```python
from build123d import *

# Parameters (mm, degrees)
SKETCH069_W                  = 20.5
SKETCH069_H                  = 15
PAD036_DEPTH                 = 1.5
SKETCH071_W                  = 0.6
SKETCH071_H                  = 0.6
PAD037_DEPTH                 = 8
SKETCH071_LINEARPATTERN_2_W  = 0.6
SKETCH071_LINEARPATTERN_2_H  = 0.6
PAD037_LINEARPATTERN_2_DEPTH = 8
SKETCH071_LINEARPATTERN_3_W  = 0.6
SKETCH071_LINEARPATTERN_3_H  = 0.6
PAD037_LINEARPATTERN_3_DEPTH = 8
SKETCH071_LINEARPATTERN_4_W  = 0.6
SKETCH071_LINEARPATTERN_4_H  = 0.6
PAD037_LINEARPATTERN_4_DEPTH = 8
SKETCH071_LINEARPATTERN_5_W  = 0.6
SKETCH071_LINEARPATTERN_5_H  = 0.6
PAD037_LINEARPATTERN_5_DEPTH = 8
SKETCH071_LINEARPATTERN_6_W  = 0.6
SKETCH071_LINEARPATTERN_6_H  = 0.6
PAD037_LINEARPATTERN_6_DEPTH = 8
SKETCH071_LINEARPATTERN_7_W  = 0.6
SKETCH071_LINEARPATTERN_7_H  = 0.6
PAD037_LINEARPATTERN_7_DEPTH = 8
SKETCH071_LINEARPATTERN_8_W  = 0.6
SKETCH071_LINEARPATTERN_8_H  = 0.6
PAD037_LINEARPATTERN_8_DEPTH = 8
SKETCH070_W                  = 20.5
SKETCH070_H                  = 2.5
PAD038_DEPTH                 = 2
SKETCH074_W                  = 1.239915
SKETCH074_H                  = 2.350915
SKETCH074_W_2                = 6.389756
SKETCH074_H_2                = 4.341472
PAD040_DEPTH                 = 0.5


with BuildPart() as part:
    # Sketch069 → Pad036 (new body)
    with BuildSketch(Plane.XY.offset(2)):
        Rectangle(SKETCH069_W, SKETCH069_H)
    extrude(amount=PAD036_DEPTH)

    # Sketch071 → Pad037 (join)
    with BuildSketch(Plane(origin=(-9.5, -6.2, 2), x_dir=(1, 0, 0), z_dir=(0, 0, 1))):
        Rectangle(SKETCH071_W, SKETCH071_H)
    pad037 = extrude(amount=-PAD037_DEPTH)

    # Sketch071 LinearPattern 2 → Pad037 LinearPattern 2 (add)
    with BuildSketch(Plane(origin=(-6.871429, -6.2, 2), x_dir=(1, 0, 0), z_dir=(0, 0, 1))):
        Rectangle(SKETCH071_LINEARPATTERN_2_W, SKETCH071_LINEARPATTERN_2_H)
    pad037_linearpattern_2 = extrude(amount=-PAD037_LINEARPATTERN_2_DEPTH)

    # Sketch071 LinearPattern 3 → Pad037 LinearPattern 3 (add)
    with BuildSketch(Plane(origin=(-4.242857, -6.2, 2), x_dir=(1, 0, 0), z_dir=(0, 0, 1))):
        Rectangle(SKETCH071_LINEARPATTERN_3_W, SKETCH071_LINEARPATTERN_3_H)
    pad037_linearpattern_3 = extrude(amount=-PAD037_LINEARPATTERN_3_DEPTH)

    # Sketch071 LinearPattern 4 → Pad037 LinearPattern 4 (add)
    with BuildSketch(Plane(origin=(-1.614286, -6.2, 2), x_dir=(1, 0, 0), z_dir=(0, 0, 1))):
        Rectangle(SKETCH071_LINEARPATTERN_4_W, SKETCH071_LINEARPATTERN_4_H)
    pad037_linearpattern_4 = extrude(amount=-PAD037_LINEARPATTERN_4_DEPTH)

    # Sketch071 LinearPattern 5 → Pad037 LinearPattern 5 (add)
    with BuildSketch(Plane(origin=(1.014286, -6.2, 2), x_dir=(1, 0, 0), z_dir=(0, 0, 1))):
        Rectangle(SKETCH071_LINEARPATTERN_5_W, SKETCH071_LINEARPATTERN_5_H)
    pad037_linearpattern_5 = extrude(amount=-PAD037_LINEARPATTERN_5_DEPTH)

    # Sketch071 LinearPattern 6 → Pad037 LinearPattern 6 (add)
    with BuildSketch(Plane(origin=(3.642857, -6.2, 2), x_dir=(1, 0, 0), z_dir=(0, 0, 1))):
        Rectangle(SKETCH071_LINEARPATTERN_6_W, SKETCH071_LINEARPATTERN_6_H)
    pad037_linearpattern_6 = extrude(amount=-PAD037_LINEARPATTERN_6_DEPTH)

    # Sketch071 LinearPattern 7 → Pad037 LinearPattern 7 (add)
    with BuildSketch(Plane(origin=(6.271429, -6.2, 2), x_dir=(1, 0, 0), z_dir=(0, 0, 1))):
        Rectangle(SKETCH071_LINEARPATTERN_7_W, SKETCH071_LINEARPATTERN_7_H)
    pad037_linearpattern_7 = extrude(amount=-PAD037_LINEARPATTERN_7_DEPTH)

    # Sketch071 LinearPattern 8 → Pad037 LinearPattern 8 (add)
    with BuildSketch(Plane(origin=(8.9, -6.2, 2), x_dir=(1, 0, 0), z_dir=(0, 0, 1))):
        Rectangle(SKETCH071_LINEARPATTERN_8_W, SKETCH071_LINEARPATTERN_8_H)
    pad037_linearpattern_8 = extrude(amount=-PAD037_LINEARPATTERN_8_DEPTH)

    # Mirrored: Pad037, Pad037 LinearPattern 2, Pad037 LinearPattern 3, Pad037 LinearPattern 4, Pad037 LinearPattern 5, Pad037 LinearPattern 6, Pad037 LinearPattern 7, Pad037 LinearPattern 8 across XZ
    add(pad037.mirror(Plane.XZ))
    add(pad037_linearpattern_2.mirror(Plane.XZ))
    add(pad037_linearpattern_3.mirror(Plane.XZ))
    add(pad037_linearpattern_4.mirror(Plane.XZ))
    add(pad037_linearpattern_5.mirror(Plane.XZ))
    add(pad037_linearpattern_6.mirror(Plane.XZ))
    add(pad037_linearpattern_7.mirror(Plane.XZ))
    add(pad037_linearpattern_8.mirror(Plane.XZ))

    # Sketch070 → Pad038 (join)
    with BuildSketch(Plane.XY.offset(2)):
        with Locations((0, 6.25)):
            Rectangle(SKETCH070_W, SKETCH070_H)
        with Locations((0, -6.25)):
            Rectangle(SKETCH070_W, SKETCH070_H)
    extrude(amount=-PAD038_DEPTH)

    # Sketch074 → Pad040 (join)
    with BuildSketch(Plane.XY.offset(3.5)):
        with Locations((-9.283549, -5.743839)):
            Rectangle(SKETCH074_W, SKETCH074_H)
        Rectangle(SKETCH074_W_2, SKETCH074_H_2)
    extrude(amount=PAD040_DEPTH)


solid = part.part
```
Can you work these out from the model? Positions are in its coordinate system, mm. A direction names the side the tool comes from. Give positions to 0.01 mm unless a question says otherwise; leave off trailing zeros. Loops run counter-clockwise (first coordinate to the right, second up) from the corner with the lowest first, then second, coordinate; pieces in that order, holes last. Notation, with made-up numbers: M 8.25,44 L 29.25,44 A22 cw 29.25,82 Z; hole C 29.25,-26.5 d11. An arc over 180 degrees is marked long. Answer in a Markdown table with one row per item.
1. Suppose I cut it at D-D on z = -0.75. Count the separate pieces of the cut face and the enclosed holes in it, plus the area to 3 significant figures.
Taken from the geometry:
| item | result |
|---|---|
| separate pieces | 16 |
| enclosed holes | 0 |
| area | 5.76 mm² |
2. If I drill on line 1 along Y through (x, z) = (0.75, -0.5); line 2 along Y through (x, z) = (8.5, 1.25); line 3 along Z through (x, y) = (-8.5, 6.25), over which ranges is the centre line in solid material (lowest first)?
Taken from the geometry:
| item | result |
|---|---|
| line 1 | y = -6.5 to -5.9, 5.9 to 6.5 |
| line 2 | y = -7.5 to -5, 5 to 7.5 |
| line 3 | z = 0 to 3.5 |
3. Thinking about a two-plate mould opening in Y: for faces 3 (the flat face through (0, 0, 4)), 4 (the flat face through (0, 7.5, 2)), 5 (the flat face through (0, 0, 2)), 6 (the flat face through (0, -7.5, 2)), which applies, released by +Y, released by -Y, zero draft, split by the parting line, or undercut?
Taken from the geometry:
| item | result |
|---|---|
| face 3 | zero draft |
| face 4 | released by +Y |
| face 5 | undercut |
| face 6 | released by -Y |
4. Suppose I cut it at B-B on x = -2.75. Write out the boundary of the cut face in (y, z), plus the area to 3 significant figures.
Taken from the geometry:
| item | result |
|---|---|
| outline | M -7.5,0 L -5,0 L -5,2 L 5,2 L 5,0 L 7.5,0 L 7.5,3.5 L 2.17,3.5 L 2.17,4 L -2.17,4 L -2.17,3.5 L -7.5,3.5 Z |
| area | 34.7 mm² |
5. Which directions (+Z, -Z, +X, -X, +Y, -Y) give clear straight access to the entire face, cutting with the end or side of a thin tool? Please do faces 1 (the flat face through (-9, -6, 4)), 2 (the flat face through (0, 5, 1)).
Taken from the geometry:
| item | result |
|---|---|
| face 1 | +Z, +X, -X, +Y, -Y |
| face 2 | -Z, +X, -X |
6. Suppose I cut it at A-A on z = 0.25. Write out the boundary of the cut face in (x, y), plus the area to 4 significant figures.
Taken from the geometry:
| item | result |
|---|---|
| outline | M -10.25,-7.5 L 10.25,-7.5 L 10.25,-5 L -10.25,-5 Z; M -10.25,5 L 10.25,5 L 10.25,7.5 L -10.25,7.5 Z |
| area | 102.5 mm² |
7. Suppose I cut it at C-C on y = 1. Write out the boundary of the cut face in (x, z).
Taken from the geometry:
| item | result |
|---|---|
| outline | M -10.25,2 L 10.25,2 L 10.25,3.5 L 3.19,3.5 L 3.19,4 L -3.19,4 L -3.19,3.5 L -10.25,3.5 Z |
8. For pin 1 Ø0.5 at (x, z) = (6.5, -3) entering from +Y; pin 2 Ø0.7 at (y, z) = (-6, -4.5) entering from -X; pin 3 Ø0.7 at (y, z) = (-6, -2) entering from +X, each with a flat end and sliding along its axis, tell me the tip position at first contact or that it passes through.
Taken from the geometry:
| item | result |
|---|---|
| pin 1 | stops at y = 6.5 |
| pin 2 | stops at x = -9.8 |
| pin 3 | stops at x = 9.2 |
